Check sheet for the modelled part. Datum: model origin and axes. Units: mm. A direction names the side the tool comes from. Round coordinates to 2 decimals unless told otherwise and drop trailing zeros. Write each loop counter-clockwise with the first axis right and the second up, starting at its lowest first coordinate (ties: lowest second). Pieces come first, ordered by that corner, then holes. Notation, with made-up numbers: (20, 72) - (64, 72) arc R23 cw to (64, 91) - close; hole circle Ø7 at (-31, 26.25). An arc over 180 degrees is marked (long way). Use one line per item in the form item = value. Start each with the question number.
1) Scan lines: probe 1 along Z at (x, y) = (1, 1.05); probe 2 along Y at (x, z) = (2, -2.75); probe 3 along Z at (x, y) = (4, 0.8). Record each from-to range of solid material in increasing order.
2) Set-up check for faces 1 (the face through (0, 2, 0)), 2 (the face through (0, 0, 0)): record each of +Z, -Z, +X, -X, +Y, -Y from which the full face is reachable in a straight line by a thin tool's end or side.
3) Section check A-A (x = -0.5). Record the boundary of the cut face in (y, z).
4) Section check C-C (z = -5.5). Record the boundary of the cut face in (x, y).
5) Section check B-B (y = 0.6). Record the boundary of the cut face in (x, z).
6) Gauge pin test, flat ends, axial feed: P1, Ø0.9, axis at y = 1, z = -11.26, coming from the +X side; P2, Ø5, axis at x = -2.5, z = -3, coming from the +Y side. Record the tip position at first contact, or that the pin passes through.
7) Draft check along Z on faces 3 (the face through (0, 1, 11.738)), 4 (the face through (0.067, 1.033, -10.513)), 5 (the face through (4.75, 1, 0)). Enter one of: +Z half, -Z half, draft (parallel to the pull), parting line (faces both ways), or undercut.
from build123d import *

# Parameters (mm, degrees)
SKETCH_1_W          = 9.5
SKETCH_1_H          = 24
EXTRUDE_1_DEPTH     = 2
SKETCH_5_R          = 0.75
CUT_EXTRUDE_4_DEPTH = 10.5
EXTRUDE_2_DEPTH     = 9.5


with BuildPart() as part:
    # 草图1 → 凸台-拉伸1 (new body)
    with BuildSketch(Plane(origin=(0, 0, 0), x_dir=(1, 0, 0), z_dir=(0, 1, 0))):
        with Locations((0, 0.261859188)):
            Rectangle(SKETCH_1_W, SKETCH_1_H)
    extrude(amount=EXTRUDE_1_DEPTH)

    # 草图5 → 切除-拉伸4 (cut, through all)
    with BuildSketch(Plane(origin=(4.75, 0, 0), x_dir=(0, 0, -1), z_dir=(1, 0, 0))):
        with BuildLine():
            Line((12.261859188, 0), (12.261859188, 1))
            ThreePointArc((12.261859188, 1), (11.968965969, 0.292893219), (11.261859188, 0))
            Line((11.261859188, 0), (12.261859188, 0))
        make_face()
        with BuildLine():
            Line((11.839209457, 2), (11.761859188, 1.866025404))
            ThreePointArc((11.761859188, 1.866025404), (12.127884592, 1.5), (12.261859188, 1))
            Line((12.261859188, 1), (12.261859188, 2))
            Line((12.261859188, 2), (11.839209457, 2))
        make_face()
        with Locations((11.261859188, 1)):
            Circle(SKETCH_5_R)
    extrude(amount=-CUT_EXTRUDE_4_DEPTH, mode=Mode.SUBTRACT)

    # 草图5<4> → 凸台-拉伸2 (add)
    with BuildSketch(Plane(origin=(4.75, 0, 0), x_dir=(0, 0, -1), z_dir=(1, 0, 0))):
        Polygon((11.261859188, 2), (11.839209457, 2), (11.884340006, 2.078168404), (11.269731653, 2.433012702), (11.019731653, 2), align=None)
    extrude(amount=-EXTRUDE_2_DEPTH)


solid = part.part
Results are:
q1.probe_1 = -12.26 to -12.01, -10.51 to 11.74
q1.probe_2 = 0 to 2
q1.probe_3 = -12.24 to -11.98, -10.54 to 11.74
q2.face_1 = +Z, +X, -X, +Y
q2.face_2 = +Z, -Z, +X, -X, -Y
q3.outline = (0, -11.26) arc R1 ccw to (1.87, -11.76) - (2.08, -11.88) - (2.43, -11.27) - (2, -11.02) - (2, 11.74) - (0, 11.74) - close; hole circle Ø1.5 at (1, -11.26)
q4.outline = (-4.75, 0) - (4.75, 0) - (4.75, 2) - (-4.75, 2) - close
q5.outline = (-4.75, -12.18) - (4.75, -12.18) - (4.75, -11.9) - (-4.75, -11.9) - close; (-4.75, -10.63) - (4.75, -10.63) - (4.75, 11.74) - (-4.75, 11.74) - close
q6.P1 = through
q6.P2 = 2
q7.face_3 = +Z half
q7.face_4 = undercut
q7.face_5 = draft
